```python
from build123d import *

# Parameters (mm, degrees)
BOSS_EXTRUDE1_DEPTH  = 39.5
CUT_EXTRUDE1_DEPTH   = 75.75264493648368
M7_CLEARANCE_HOLE1_D = 8
FILLET1_R            = 10
FILLET3_R            = 2
BOSS_EXTRUDE2_REACH  = 76.753
SKETCH3_3_R          = 9.724999999999993
SKETCH3_3_R_2        = 4.4


with BuildPart() as part:
    # Sketch2 → Boss-Extrude1 (new body)
    with BuildSketch(Plane.XY):
        with BuildLine():
            Line((-15.914999999999996, 0), (-15.914999999999988, -54.904999999999994))
            Line((-15.914999999999988, -54.904999999999994), (-12.514999999999986, -54.904999999999994))
            Line((-12.514999999999986, -54.904999999999994), (-12.515, -25))
            ThreePointArc((-12.515, -25), (4.71e-15, -33.47684031960013), (12.515, -25))
            Line((12.515, -25), (12.515000000000002, -54.904999999999994))
            Line((12.515000000000002, -54.904999999999994), (15.915, -54.904999999999994))
            Line((15.915, -54.904999999999994), (15.914999999999996, 3.9e-15))
            ThreePointArc((15.914999999999996, 3.9e-15), (9.7e-16, 15.914999999999996), (-15.914999999999996, 0))
        make_face()
        with BuildLine():
            Line((10.3, 1.26e-15), (10.3, -17.7))
            ThreePointArc((10.3, -17.7), (3.82e-15, -28), (-10.299999999999997, -17.700000000000003))
            Line((-10.299999999999997, -17.700000000000003), (-10.3, -1.26e-15))
            ThreePointArc((-10.3, -1.26e-15), (-1.66e-15, 10.3), (10.3, 1.26e-15))
        make_face(mode=Mode.SUBTRACT)
    extrude(amount=BOSS_EXTRUDE1_DEPTH)

    # Sketch3 → Cut-Extrude1 (cut, through all)
    with BuildSketch(Plane.ZY.offset(15.914999999999996)):
        with BuildLine():
            Line((0, -54.904999999999994), (19.74999999999999, -54.904999999999994))
            ThreePointArc((19.74999999999999, -54.904999999999994), (12.873386552960827, -52.05661344703917), (10.025000000000007, -45.18))
            Line((10.025, -45.18), (0, -33.47684031960014))
            Line((0, -33.47684031960014), (0, -54.904999999999994))
        make_face()
        with BuildLine():
            Line((19.74999999999999, -54.904999999999994), (39.5, -54.904999999999994))
            Line((39.5, -54.904999999999994), (39.5, -33.47684031960014))
            Line((39.5, -33.47684031960014), (29.475, -45.18))
            ThreePointArc((29.474999999999994, -45.18), (26.626613447039162, -52.056613447039176), (19.74999999999999, -54.904999999999994))
        make_face()
    extrude(amount=-CUT_EXTRUDE1_DEPTH, mode=Mode.SUBTRACT)

    # M7 Clearance Hole1 (through all)
    with Locations(Plane.ZY.offset(15.914999999999996)):
        with Locations((19.75, -45.18)):
            Hole(M7_CLEARANCE_HOLE1_D / 2)

    # Fillet1
    fillet1_edges = [part.edges().sort_by_distance(p)[0] for p in [
        (-14.21499999999999, -45.18, 10.025000000000002),
        (14.215000000000002, -45.17999999999999, 10.025000000000002),
        (-14.214999999999993, -33.47684031960014, 0),
        (14.215, -33.476840319600136, 0),
        (-14.21499999999999, -45.18, 29.474999999999998),
        (14.215000000000002, -45.17999999999999, 29.474999999999998),
        (-14.214999999999993, -33.47684031960014, 39.5),
        (14.215, -33.476840319600136, 39.5),
    ]]
    fillet(fillet1_edges, radius=FILLET1_R)

    # Fillet3
    fillet3_edges = [part.edges().sort_by_distance(p)[0] for p in [
        (12.515, -25, 19.75),
        (-12.515000000000002, -25, 19.75),
    ]]
    fillet(fillet3_edges, radius=FILLET3_R)

    # Boss-Extrude2: up to this face of the body (flat: up to its plane)
    boss_extrude2_end = Plane(part.part.faces().sort_by_distance((12.515, -40.102126489, 19.75))[0])
    # Sketch3<3> → Boss-Extrude2 (add, up to the picked face)
    with BuildSketch(Plane.ZY.offset(15.914999999999996), mode=Mode.PRIVATE) as boss_extrude2_sk1:
        with Locations((19.75, -45.18)):
            Circle(SKETCH3_3_R)
        with Locations(Location((19.75, -45.18, 0), (0, 0, 270))):
            Circle(SKETCH3_3_R_2, mode=Mode.SUBTRACT)
    boss_extrude2_tool1 = split(extrude(boss_extrude2_sk1.sketch, amount=-BOSS_EXTRUDE2_REACH, mode=Mode.PRIVATE), bisect_by=boss_extrude2_end, keep=Keep.BOTH, mode=Mode.PRIVATE)
    # Sketch3<3> → Boss-Extrude2 (add, up to the picked face)
    with BuildSketch(Plane.ZY.offset(15.914999999999996), mode=Mode.PRIVATE) as boss_extrude2_sk2:
        with BuildLine():
            Line((17.206534975176847, -35.77037402891417), (17.293465024823192, -35.77037402891417))
            ThreePointArc((17.293465024823192, -35.77037402891417), (19.750000000000018, -35.455000000000005), (22.206534975176844, -35.770374028914176))
            Line((22.206534975176847, -35.77037402891417), (22.206534975176847, -28.83040215808249))
            ThreePointArc((22.20653497517679, -28.830402158082467), (19.697179052869707, -29.57968293716084), (17.20653497517685, -28.770374028914166))
            Line((17.206534975176847, -28.77037402891417), (17.206534975176847, -35.77037402891417))
        make_face()
    boss_extrude2_tool2 = split(extrude(boss_extrude2_sk2.sketch, amount=-BOSS_EXTRUDE2_REACH, mode=Mode.PRIVATE), bisect_by=boss_extrude2_end, keep=Keep.BOTH, mode=Mode.PRIVATE)
    # Sketch3<3> → Boss-Extrude2 (add, up to the picked face)
    with BuildSketch(Plane.ZY.offset(15.914999999999996), mode=Mode.PRIVATE) as boss_extrude2_sk3:
        with BuildLine():
            ThreePointArc((22.206534975176844, -35.770374028914176), (19.750000000000018, -35.455000000000005), (17.293465024823192, -35.77037402891417))
            Line((17.293465024823192, -35.77037402891417), (22.206534975176847, -35.77037402891417))
        make_face()
    boss_extrude2_tool3 = split(extrude(boss_extrude2_sk3.sketch, amount=-BOSS_EXTRUDE2_REACH, mode=Mode.PRIVATE), bisect_by=boss_extrude2_end, keep=Keep.BOTH, mode=Mode.PRIVATE)
    add(boss_extrude2_tool1.solids().sort_by(Axis((-15.915, -45.18, 10.300065), (1, 1.9e-16, 0)))[0])
    add(boss_extrude2_tool2.solids().sort_by(Axis((-15.915, -32.443059, 19.701397), (1, 1.9e-16, 0)))[0])
    add(boss_extrude2_tool3.solids().sort_by(Axis((-15.915, -35.644047, 19.75), (1, 1.9e-16, 0)))[0])


solid = part.part
```
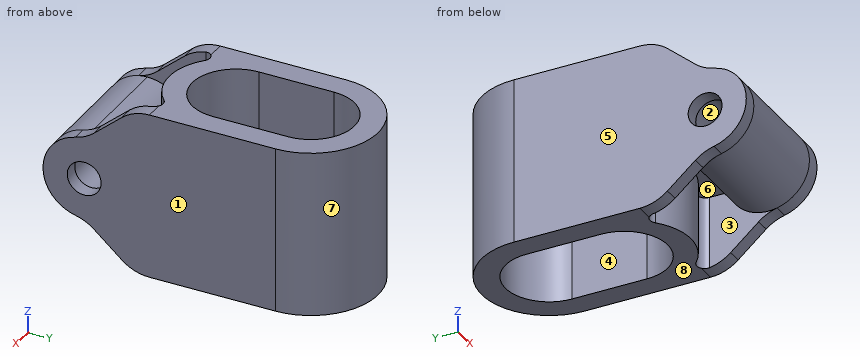
Build history of the part. All positions in model axes, mm. Face numbers are marked on the shaded views. A direction names the side the tool comes from. Round coordinates to 2 decimals unless told otherwise and drop trailing zeros. Write each loop counter-clockwise with the first axis right and the second up, starting at its lowest first coordinate (ties: lowest second). Pieces come first, ordered by that corner, then holes. Notation, with made-up numbers: (-16, -0.5) -> (-1, -0.5) arc R20 cw to (-1, 16.5) -> close; hole circle Ø1 at (23, -24). An arc over 180 degrees is marked (long way). Put each result on its own line as item: value.
Item 1: Two-plate mould, pull along X, no slides. Class the marked faces 5, 6, 7 and 8: pulls with the +X half, pulls with the -X half, needs draft (parallel to the pull), parting line crosses it, or undercut.
Here are the results:
face 5: pulls with the -X half
face 6: undercut
face 7: parting line crosses it
face 8: needs draft
Item 2: Slice it at A-A, the plane z = 19.75. Give the cut face in (x, y) (3 decimals).
Here are the results:
outline: (-15.915, -54.905) -> (15.915, -54.905) -> (15.915, -49.18) -> (12.515, -49.18) -> (12.515, -49.58) -> (-12.515, -49.58) -> (-12.515, -49.18) -> (-15.915, -49.18) -> close; (-15.915, -41.18) -> (-12.515, -41.18) -> (-12.515, -40.78) -> (12.515, -40.78) -> (12.515, -41.18) -> (15.915, -41.18) -> (15.915, 0) arc R15.915 ccw to (-15.915, 0) -> close; hole (-11.434, -29.58) -> (-9.596, -29.58) arc R2 ccw to start; hole (-10.3, -17.7) arc R10.3 ccw to (10.3, -17.7) -> (10.3, 0) arc R10.3 ccw to (-10.3, 0) -> close; hole (9.596, -29.58) -> (11.434, -29.58) arc R2 ccw to start
Item 3: Flat gauge pins, fed straight in: P1, Ø5, axis at x = -7.5, z = 21.5, coming from the -Y side (3 decimals); P2, Ø1.5, axis at x = -10.5, z = 25.5, coming from the +Y side; P3, Ø3, axis at y = 3.5, z = 15.5, coming from the +X side; P4, Ø8, axis at x = -0.5, z = 32.5, coming from the -Y side. Where does each tip first touch, or does it go through?
Here are the results:
P1: stops at y = -54.905
P2: stops at y = 12.58
P3: stops at x = 15.79
P4: stops at y = -49.42
Item 4: Wall check: probe 1 along X at (y, z) = (-36.5, 35) (3 decimals); probe 2 along Z at (x, y) = (-5.25, -45.18) (3 decimals); probe 3 along X at (y, z) = (-1.5, 7) (3 decimals). Give the ranges that are in metal, low to high. Write a range as from..to.
Here are the results:
probe 1: x = -15.915..-12.515, 12.515..15.915
probe 2: z = 10.025..15.35, 24.15..29.475
probe 3: x = -15.915..-10.3, 10.3..15.915
Item 5: Tool access for the marked faces 1, 2, 3 and 4: list every direction of +Z, -Z, +X, -X, +Y, -Y with a clear straight run to the whole face (end or side of a thin tool).
Here are the results:
face 1: +Z, -Z, +X, +Y, -Y
face 2: none
face 3: -Z
face 4: +Z, -Z
Item 6: Slice it at C-C, the plane x = 0. Give the cut face in (y, z) (3 decimals).
Here are the results:
outline: (-35.77, 17.207) -> (-33.477, 17.207) -> (-33.477, 0) -> (-28, 0) -> (-28, 39.5) -> (-33.477, 39.5) -> (-33.477, 22.207) -> (-35.77, 22.207) arc R9.725 ccw (long way) to (-35.77, 17.293) -> close; (10.3, 0) -> (15.915, 0) -> (15.915, 39.5) -> (10.3, 39.5) -> close; hole circle Ø8.8 at (-45.18, 19.75)
Item 7: Slice it at B-B, the plane y = -16. Give the cut face in (x, z) (3 decimals), plus the area to 3 significant figures.
Here are the results:
outline: (-15.915, 0) -> (-10.3, 0) -> (-10.3, 39.5) -> (-15.915, 39.5) -> close; (10.3, 0) -> (15.915, 0) -> (15.915, 39.5) -> (10.3, 39.5) -> close
area: 444 mm^2
Item 8: Slice it at D-D, the plane x = 6.5. Give the cut face in (y, z) (3 decimals), plus the area to 3 significant figures.
Here are the results:
outline: (-35.77, 17.207) -> (-31.806, 17.207) -> (-31.806, 0) -> (-25.69, 0) -> (-25.69, 39.5) -> (-31.806, 39.5) -> (-31.806, 22.207) -> (-35.77, 22.207) arc R9.725 ccw (long way) to (-35.77, 17.293) -> close; (7.99, 0) -> (14.527, 0) -> (14.527, 39.5) -> (7.99, 39.5) -> close; hole circle Ø8.8 at (-45.18, 19.75)
area: 755 mm^2
